Build history of the part. All positions in model axes, mm. A direction names the side the tool comes from. Give positions to 0.01 mm unless a question says otherwise; leave off trailing zeros. Order: outer loops, then holes, each group sorted by start corner. A loop starts at its lowest first (then second) coordinate and runs counter-clockwise, first axis right, second up. Notation, with made-up numbers: (62.5, 70) - (70.5, 70) arc R17 cw to (70.5, 91) - close; hole circle Ø5 at (48, 5.5). An arc over 180 degrees is marked (long way). Use a Markdown table: item, result.
from build123d import *

# Parameters (mm, degrees)
F0_W     = 120
F0_H     = 90
F0_R     = 2.25
F0_R_2   = 5.25
F1_DEPTH = 25
F2_R     = 2.25
F2_R_2   = 5.25
F3_DEPTH = 16
F4_R     = 5.25
F4_R_2   = 2.25
F5_DEPTH = 3
F6_R     = 2.25
F7_DEPTH = 9.001


with BuildPart() as f1:
    # F0 (on Front) → F1 (new body)
    with BuildSketch(Plane.XZ):
        Rectangle(F0_W, F0_H)
        with BuildLine():
            Line((-43, 30), (43, 30))
            ThreePointArc((43, 30), (44.4142135624, 29.4142135624), (45, 28))
            Line((45, 28), (45, -28))
            ThreePointArc((45, -28), (44.4142135624, -29.4142135624), (43, -30))
            Line((43, -30), (-43, -30))
            ThreePointArc((-43, -30), (-44.4142135624, -29.4142135624), (-45, -28))
            Line((-45, -28), (-45, 28))
            ThreePointArc((-45, 28), (-44.4142135624, 29.4142135624), (-43, 30))
        make_face(mode=Mode.SUBTRACT)
        with BuildLine():
            ThreePointArc((45, 28), (44.4142135624, 29.4142135624), (43, 30))
            Line((43, 30), (-43, 30))
            ThreePointArc((-43, 30), (-44.4142135624, 29.4142135624), (-45, 28))
            Line((-45, 28), (-45, -28))
            ThreePointArc((-45, -28), (-44.4142135624, -29.4142135624), (-43, -30))
            Line((-43, -30), (43, -30))
            ThreePointArc((43, -30), (44.4142135624, -29.4142135624), (45, -28))
            Line((45, -28), (45, 28))
        make_face()
        with Locations((25, -15)):
            Circle(F0_R, mode=Mode.SUBTRACT)
        with Locations((-25, 15)):
            Circle(F0_R_2, mode=Mode.SUBTRACT)
        with BuildLine():
            Line((1.5, 1.5), (6, 1.5))
            ThreePointArc((6, 1.5), (7.0606601718, 1.0606601718), (7.5, 0))
            ThreePointArc((7.5, 0), (7.0606601718, -1.0606601718), (6, -1.5))
            Line((6, -1.5), (1.5, -1.5))
            Line((1.5, -1.5), (1.5, -6))
            ThreePointArc((1.5, -6), (1.0606601718, -7.0606601718), (0, -7.5))
            ThreePointArc((0, -7.5), (-1.0606601718, -7.0606601718), (-1.5, -6))
            Line((-1.5, -6), (-1.5, -1.5))
            Line((-1.5, -1.5), (-6, -1.5))
            ThreePointArc((-6, -1.5), (-7.0606601718, -1.0606601718), (-7.5, 0))
            ThreePointArc((-7.5, 0), (-7.0606601718, 1.0606601718), (-6, 1.5))
            Line((-6, 1.5), (-1.5, 1.5))
            Line((-1.5, 1.5), (-1.5, 6))
            ThreePointArc((-1.5, 6), (-1.0606601718, 7.0606601718), (0, 7.5))
            ThreePointArc((0, 7.5), (1.0606601718, 7.0606601718), (1.5, 6))
            Line((1.5, 6), (1.5, 1.5))
        make_face(mode=Mode.SUBTRACT)
        with Locations((-25, 15)):
            Circle(F0_R_2)
        with Locations((-25, 15)):
            Circle(F0_R, mode=Mode.SUBTRACT)
        with BuildLine():
            ThreePointArc((7.5, 0), (7.0606601718, 1.0606601718), (6, 1.5))
            Line((6, 1.5), (1.5, 1.5))
            Line((1.5, 1.5), (1.5, 6))
            ThreePointArc((1.5, 6), (1.0606601718, 7.0606601718), (0, 7.5))
            ThreePointArc((0, 7.5), (-1.0606601718, 7.0606601718), (-1.5, 6))
            Line((-1.5, 6), (-1.5, 1.5))
            Line((-1.5, 1.5), (-6, 1.5))
            ThreePointArc((-6, 1.5), (-7.0606601718, 1.0606601718), (-7.5, 0))
            ThreePointArc((-7.5, 0), (-7.0606601718, -1.0606601718), (-6, -1.5))
            Line((-6, -1.5), (-1.5, -1.5))
            Line((-1.5, -1.5), (-1.5, -6))
            ThreePointArc((-1.5, -6), (-1.0606601718, -7.0606601718), (0, -7.5))
            ThreePointArc((0, -7.5), (1.0606601718, -7.0606601718), (1.5, -6))
            Line((1.5, -6), (1.5, -1.5))
            Line((1.5, -1.5), (6, -1.5))
            ThreePointArc((6, -1.5), (7.0606601718, -1.0606601718), (7.5, 0))
        make_face()
        with Locations((-25, 15)):
            Circle(F0_R)
        with Locations((25, -15)):
            Circle(F0_R)
    extrude(amount=-F1_DEPTH)

    # F2 (on face) → F3 (cut)
    with BuildSketch(Plane.XZ):
        with BuildLine():
            ThreePointArc((45.579787234, 27.6010638298), (44.9940007964, 29.0152773922), (43.579787234, 29.6010638298))
            Line((43.579787234, 29.6010638298), (-42.420212766, 29.6010638298))
            ThreePointArc((-42.420212766, 29.6010638298), (-43.8344263283, 29.0152773922), (-44.420212766, 27.6010638298))
            Line((-44.420212766, 27.6010638298), (-44.420212766, -28.3989361702))
            ThreePointArc((-44.420212766, -28.3989361702), (-43.8344263283, -29.8131497326), (-42.420212766, -30.3989361702))
            Line((-42.420212766, -30.3989361702), (43.579787234, -30.3989361702))
            ThreePointArc((43.579787234, -30.3989361702), (44.9940007964, -29.8131497326), (45.579787234, -28.3989361702))
            Line((45.579787234, -28.3989361702), (45.579787234, 27.6010638298))
        make_face()
        with Locations((25.579787234, -15.3989361702)):
            Circle(F2_R, mode=Mode.SUBTRACT)
        with BuildLine():
            Line((2.079787234, 1.1010638298), (6.579787234, 1.1010638298))
            ThreePointArc((6.579787234, 1.1010638298), (7.6404474058, 0.6617240016), (8.079787234, -0.3989361702))
            ThreePointArc((8.079787234, -0.3989361702), (7.6404474058, -1.459596342), (6.579787234, -1.8989361702))
            Line((6.579787234, -1.8989361702), (2.079787234, -1.8989361702))
            Line((2.079787234, -1.8989361702), (2.079787234, -6.3989361702))
            ThreePointArc((2.079787234, -6.3989361702), (1.6404474058, -7.459596342), (0.579787234, -7.8989361702))
            ThreePointArc((0.579787234, -7.8989361702), (-0.4808729377, -7.459596342), (-0.920212766, -6.3989361702))
            Line((-0.920212766, -6.3989361702), (-0.920212766, -1.8989361702))
            Line((-0.920212766, -1.8989361702), (-5.420212766, -1.8989361702))
            ThreePointArc((-5.420212766, -1.8989361702), (-6.4808729377, -1.459596342), (-6.920212766, -0.3989361702))
            ThreePointArc((-6.920212766, -0.3989361702), (-6.4808729377, 0.6617240016), (-5.420212766, 1.1010638298))
            Line((-5.420212766, 1.1010638298), (-0.920212766, 1.1010638298))
            Line((-0.920212766, 1.1010638298), (-0.920212766, 5.6010638298))
            ThreePointArc((-0.920212766, 5.6010638298), (-0.4808729377, 6.6617240016), (0.579787234, 7.1010638298))
            ThreePointArc((0.579787234, 7.1010638298), (1.6404474058, 6.6617240016), (2.079787234, 5.6010638298))
            Line((2.079787234, 5.6010638298), (2.079787234, 1.1010638298))
        make_face(mode=Mode.SUBTRACT)
        with Locations((-24.420212766, 14.6010638298)):
            Circle(F2_R_2, mode=Mode.SUBTRACT)
        with Locations((-24.420212766, 14.6010638298)):
            Circle(F2_R_2)
        with Locations((-24.420212766, 14.6010638298)):
            Circle(F2_R, mode=Mode.SUBTRACT)
        with Locations((-24.420212766, 14.6010638298)):
            Circle(F2_R)
        with BuildLine():
            ThreePointArc((8.079787234, -0.3989361702), (7.6404474058, 0.6617240016), (6.579787234, 1.1010638298))
            Line((6.579787234, 1.1010638298), (2.079787234, 1.1010638298))
            Line((2.079787234, 1.1010638298), (2.079787234, 5.6010638298))
            ThreePointArc((2.079787234, 5.6010638298), (1.6404474058, 6.6617240016), (0.579787234, 7.1010638298))
            ThreePointArc((0.579787234, 7.1010638298), (-0.4808729377, 6.6617240016), (-0.920212766, 5.6010638298))
            Line((-0.920212766, 5.6010638298), (-0.920212766, 1.1010638298))
            Line((-0.920212766, 1.1010638298), (-5.420212766, 1.1010638298))
            ThreePointArc((-5.420212766, 1.1010638298), (-6.4808729377, 0.6617240016), (-6.920212766, -0.3989361702))
            ThreePointArc((-6.920212766, -0.3989361702), (-6.4808729377, -1.459596342), (-5.420212766, -1.8989361702))
            Line((-5.420212766, -1.8989361702), (-0.920212766, -1.8989361702))
            Line((-0.920212766, -1.8989361702), (-0.920212766, -6.3989361702))
            ThreePointArc((-0.920212766, -6.3989361702), (-0.4808729377, -7.459596342), (0.579787234, -7.8989361702))
            ThreePointArc((0.579787234, -7.8989361702), (1.6404474058, -7.459596342), (2.079787234, -6.3989361702))
            Line((2.079787234, -6.3989361702), (2.079787234, -1.8989361702))
            Line((2.079787234, -1.8989361702), (6.579787234, -1.8989361702))
            ThreePointArc((6.579787234, -1.8989361702), (7.6404474058, -1.459596342), (8.079787234, -0.3989361702))
        make_face()
        with Locations((25.579787234, -15.3989361702)):
            Circle(F2_R)
    extrude(amount=-F3_DEPTH, mode=Mode.SUBTRACT)

    # F4 (on face) → F5 (cut)
    with BuildSketch(Plane.XZ.offset(-16)):
        with Locations((-23.8404255319, 14.2021276596)):
            Circle(F4_R)
        with Locations((-23.8404255319, 14.2021276596)):
            Circle(F4_R_2, mode=Mode.SUBTRACT)
    extrude(amount=-F5_DEPTH, mode=Mode.SUBTRACT)

    # F6 (on face) → F7 (cut, through all)
    with BuildSketch(Plane.XZ.offset(-16)):
        with BuildLine():
            ThreePointArc((9.0577965574, -1.0359728926), (8.6184567292, 0.0246872792), (7.5577965574, 0.4640271074))
            Line((7.5577965574, 0.4640271074), (3.0577965574, 0.4640271074))
            Line((3.0577965574, 0.4640271074), (3.0577965574, 4.9640271074))
            ThreePointArc((3.0577965574, 4.9640271074), (2.6184567292, 6.0246872792), (1.5577965574, 6.4640271074))
            ThreePointArc((1.5577965574, 6.4640271074), (0.4971363856, 6.0246872792), (0.0577965574, 4.9640271074))
            Line((0.0577965574, 4.9640271074), (0.0577965574, 0.4640271074))
            Line((0.0577965574, 0.4640271074), (-4.4422034426, 0.4640271074))
            ThreePointArc((-4.4422034426, 0.4640271074), (-5.5028636144, 0.0246872792), (-5.9422034426, -1.0359728926))
            ThreePointArc((-5.9422034426, -1.0359728926), (-5.5028636144, -2.0966330644), (-4.4422034426, -2.5359728926))
            Line((-4.4422034426, -2.5359728926), (0.0577965574, -2.5359728926))
            Line((0.0577965574, -2.5359728926), (0.0577965574, -7.0359728926))
            ThreePointArc((0.0577965574, -7.0359728926), (0.4971363856, -8.0966330644), (1.5577965574, -8.5359728926))
            ThreePointArc((1.5577965574, -8.5359728926), (2.6184567292, -8.0966330644), (3.0577965574, -7.0359728926))
            Line((3.0577965574, -7.0359728926), (3.0577965574, -2.5359728926))
            Line((3.0577965574, -2.5359728926), (7.5577965574, -2.5359728926))
            ThreePointArc((7.5577965574, -2.5359728926), (8.6184567292, -2.0966330644), (9.0577965574, -1.0359728926))
        make_face()
        with Locations((26.5577965574, -16.0359728926)):
            Circle(F6_R)
    extrude(amount=-F7_DEPTH, mode=Mode.SUBTRACT)


solid = f1.part
1) Pin check, flat tip, straight feed: P1, Ø5, axis at x = -24.5, z = 15, coming from the -Y side. Stop position of the tip, or through.
Computed:
| item | result |
|---|---|
| P1 | stops at y = 16 |
2) Wall check: line 1 (Z direction, x = -2, y = 7.25); line 2 (X direction, y = 11, z = -8.5); line 3 (Y direction, x = -18.5, z = -27). Give the ranges that are in metal, low to high. Write a range as from..to.
Computed:
| item | result |
|---|---|
| line 1 | z = -45..-30.4, 29.6..45 |
| line 2 | x = -60..-44.42, 45.58..60 |
| line 3 | y = 16..25 |
3) Slice it at A-A (y = 14.75). Write the cut outline in (x, z).
Computed:
| item | result |
|---|---|
| outline | (-60, -45) - (60, -45) - (60, 45) - (-60, 45) - close; hole (-44.42, -28.4) arc R2 ccw to (-42.42, -30.4) - (43.58, -30.4) arc R2 ccw to (45.58, -28.4) - (45.58, 27.6) arc R2 ccw to (43.58, 29.6) - (-42.42, 29.6) arc R2 ccw to (-44.42, 27.6) - close |
4) Slice it at C-C (x = 12.5). Write the cut outline in (y, z).
Computed:
| item | result |
|---|---|
| outline | (0, -45) - (25, -45) - (25, 45) - (0, 45) - (0, 29.6) - (16, 29.6) - (16, -30.4) - (0, -30.4) - close |
5) Tool access for faces 1 (the cylindrical face through (-18.833, 17.479, 15.779)), 2 (the flat face through (5, 20, 0.464)), 3 (the flat face through (-1, 0, 31)): list every direction of +Z, -Z, +X, -X, +Y, -Y with a clear straight run to the whole face (end or side of a thin tool).
Computed:
| item | result |
|---|---|
| face 1 | -Y |
| face 2 | +Y, -Y |
| face 3 | +Z, -Z, +X, -X, -Y |
6) Slice it at B-B (z = -21). Write the cut outline in (x, y).
Computed:
| item | result |
|---|---|
| outline | (-60, 0) - (-44.42, 0) - (-44.42, 16) - (45.58, 16) - (45.58, 0) - (60, 0) - (60, 25) - (-60, 25) - close |
7) Two-plate mould, pull along Z, no slides. Class faces 4 (the cylindrical face through (27.77, 20.44, -14.14)), 5 (the cylindrical face through (-21.7, 17.5, 14.9)), 6 (the flat face through (-1, 12, 45)), 7 (the flat face through (60, 12, -1)): +Z half, -Z half, draft (parallel to the pull), parting line (faces both ways), or undercut.
Computed:
| item | result |
|---|---|
| face 4 | undercut |
| face 5 | undercut |
| face 6 | +Z half |
| face 7 | draft |
